```python
from build123d import *

# Parameters (mm, degrees)
F0_W     = 50
F0_H     = 50
F0_W_2   = 45
F0_H_2   = 45
F1_DEPTH = 250


with BuildPart() as f1:
    # F0 (on Front) → F1 (new body, symmetric)
    with BuildSketch(Plane.XZ):
        with Locations((-11.886792, 20.122862)):
            Rectangle(F0_W, F0_H)
        with Locations((-11.886792, 20.122862)):
            Rectangle(F0_W_2, F0_H_2, mode=Mode.SUBTRACT)
    extrude(amount=F1_DEPTH, both=True)


solid = f1.part
```
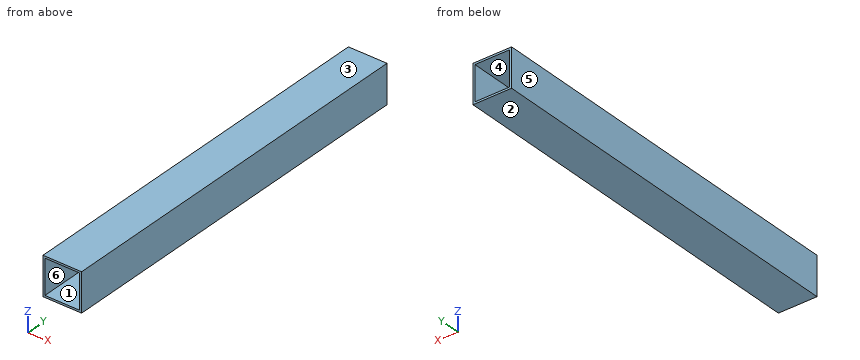
The model under review builds one solid part; all positions refer to its coordinate system, in mm. Face numbers are marked on the shaded views. A direction names the side the tool comes from. Give positions to 0.01 mm unless a question says otherwise; leave off trailing zeros. Write each loop counter-clockwise with the first axis right and the second up, starting at its lowest first coordinate (ties: lowest second). Pieces come first, ordered by that corner, then holes. Notation, with made-up numbers: (77, 37.25) -> (128, 37.25) arc R20 ccw to (128, 61.25) -> close; hole circle Ø7 at (82, 88.5). An arc over 180 degrees is marked (long way). Answer in a Markdown table with one row per item.
1) Add section A-A on z = 20.5. State the section outline as (x, y) points, plus the area to 3 significant figures.
Worked answers:
| item | result |
|---|---|
| outline | (-36.89, -250) -> (-34.39, -250) -> (-34.39, 250) -> (-36.89, 250) -> close; (10.61, -250) -> (13.11, -250) -> (13.11, 250) -> (10.61, 250) -> close |
| area | 2,500 mm² |
2) Add section C-C on x = -22. State the section outline as (y, z) points.
Worked answers:
| item | result |
|---|---|
| outline | (-250, -4.88) -> (250, -4.88) -> (250, -2.38) -> (-250, -2.38) -> close; (-250, 42.62) -> (250, 42.62) -> (250, 45.12) -> (-250, 45.12) -> close |
3) Tool access review of the marked faces 1 and 2: name each direction out of +Z, -Z, +X, -X, +Y, -Y from which nothing blocks a thin tool from reaching the whole face with its end or side.
Worked answers:
| item | result |
|---|---|
| face 1 | +Y, -Y |
| face 2 | -Z, +X, -X, +Y, -Y |
4) Add section B-B on y = -186. State the section outline as (x, z) points, plus the area to 3 significant figures.
Worked answers:
| item | result |
|---|---|
| outline | (-36.89, -4.88) -> (13.11, -4.88) -> (13.11, 45.12) -> (-36.89, 45.12) -> close; hole (-34.39, -2.38) -> (10.61, -2.38) -> (10.61, 42.62) -> (-34.39, 42.62) -> close |
| area | 475 mm² |
5) For L1, parallel to Z at x = -6, y = 164.5; L2, parallel to X at y = 198.5, z = 9, list the stretches that pass through material, from the lowest coordinate up. Write a range as [from, to].
Worked answers:
| item | result |
|---|---|
| L1 | [-4.88, -2.38], [42.62, 45.12] |
| L2 | [-36.89, -34.39], [10.61, 13.11] |
6) Mouldability with a two-part tool opening along Z and no side actions: class the marked faces 3, 4, 5 and 6 as +Z half, -Z half, draft (parallel to the pull), parting line (faces both ways), or undercut.
Worked answers:
| item | result |
|---|---|
| face 3 | +Z half |
| face 4 | undercut |
| face 5 | draft |
| face 6 | undercut |
7) Clearance check with a flat-ended pin moving along its axis: P1, Ø12, axis at x = -7, z = 38, coming from the +Y side. State where the tip first meets the part, or that it passes through.
Worked answers:
| item | result |
|---|---|
| P1 | y = 250 |
